Could you check a few things on this model? Use its own coordinates, in mm. A direction names the side the tool comes from. Give positions to 0.01 mm unless a question says otherwise; leave off trailing zeros. Loops run counter-clockwise (first coordinate to the right, second up) from the corner with the lowest first, then second, coordinate; pieces in that order, holes last. Notation, with made-up numbers: (-2, 18.5) -> (29, 18.5) arc R25 ccw to (29, 52.5) -> close; hole circle Ø7 at (25.5, 41.25). An arc over 180 degrees is marked (long way). Write each question's results on one line, items separated by ' | '. Start each with the question number.
Q1. We'd pull the mould along Z, two halves only. Please class faces 5 (the face through (12.446, 88.46, -178.465)), 6 (the face through (196, 87.7, -346.1)), 7 (the face through (-12, 177.8, -108)): released by +Z, released by -Z, zero draft, split by the parting line, or undercut.
Q2. If we section it at C-C, the plane x = 146.05: List the corners of the cut face in (y, z) for me (1 decimal).
Q3. If I drill on line 1 along Z through (x, y) = (146.05, 76) (1 decimal); line 2 along Y through (x, z) = (110, -272); line 3 along Z through (x, y) = (192.5, 96.5), over which ranges is the centre line in solid material (lowest first)?
Q4. Will these pins go through, and if not, where does the flat tip stop? P1, Ø0.8, axis at y = 40.5, z = 5.5, coming from the +X side; P2, Ø1.7, axis at x = -39, y = 40.5, coming from the +Z side (3 decimals); P3, Ø0.7, axis at y = 84, z = -36, coming from the -X side (3 decimals); P4, Ø5, axis at x = 142.5, z = -298, coming from the -Y side.
Q5. Which directions (+Z, -Z, +X, -X, +Y, -Y) give clear straight access to the entire face, cutting with the end or side of a thin tool? Please do faces 1 (the face through (64, 39.688, 25)), 2 (the face through (100, 0, -154)), 3 (the face through (-38.9, 41.275, -23.5)), 4 (the face through (-21.262, 21.153, 38.673)).
Q6. If we section it at D-D, the plane z = -306: List the corners of the cut face in (x, y) for me.
from build123d import *

# Parameters (mm, degrees)
F1_DEPTH  = 177.8
F3_T      = -1.5875
F4_W      = 201.5869445521
F4_H      = 226.8152372871
F5_DEPTH  = 137.796
F6_R      = 3.571875
F7_DEPTH  = 1.5875
F9_W      = 76.2
F9_H      = 19.05
F10_DEPTH = 154.0954613767


with BuildPart() as f1:
    # F0 (on Front) → F1 (new body)
    with BuildSketch(Plane.XZ):
        with BuildLine():
            Line((224.489292991, -184.5372190302), (34.2280551234, 30.3110316959))
            ThreePointArc((34.2280551234, 30.3110316959), (-22.7900998011, 39.6349561758), (-43.415004865, -14.3337277974))
            Line((-43.415004865, -14.3337277974), (46.5572805176, -286.8481262024))
            ThreePointArc((46.5572805176, -286.8481262024), (198.2773120441, -344.8301079029), (224.489292991, -184.5372190302))
        make_face()
    extrude(amount=-F1_DEPTH)

    # F3
    f3_openings = [f1.faces().sort_by_distance(p)[0] for p in [
        (100.456199, 177.8, -174.706432),
    ]]
    offset(amount=F3_T, openings=f3_openings)

    # F4 (on offset) → F5 (cut, through all)
    with BuildSketch(Plane.YZ.offset(92.075)):
        with Locations((142.068472276, 21.3326186436)):
            Rectangle(F4_W, F4_H)
    extrude(amount=-F5_DEPTH, mode=Mode.SUBTRACT)

    # F6 (on face) → F7 (join)
    with BuildSketch(Plane(origin=(0, 41.275, 0), x_dir=(-1, 0, 0), z_dir=(0, 1, 0))):
        with BuildLine():
            Line((-13.52243099, 42.0097776282), (-80.9625, 41.275))
            Line((-80.9625, 41.275), (-80.9625, -24.8573199515))
            Line((-80.9625, -24.8573199515), (-33.0395809871, 29.2585653176))
            ThreePointArc((-33.0395809871, 29.2585653176), (-24.1382185276, 36.9462306949), (-13.52243099, 42.0097776282))
        make_face()
        with Locations((-71.4375, 22.47392)):
            Circle(F6_R, mode=Mode.SUBTRACT)
        with BuildLine():
            Line((80.9625, -73.025), (80.9625, 41.275))
            Line((80.9625, 41.275), (15.6221615422, 41.275))
            ThreePointArc((15.6221615422, 41.275), (39.833691772, 18.9988040694), (41.9075394183, -13.8360289155))
            Line((41.9075394183, -13.8360289155), (22.3659407759, -73.025))
            Line((22.3659407759, -73.025), (80.9625, -73.025))
        make_face()
        with Locations((71.4375, -53.72608)):
            Circle(F6_R, mode=Mode.SUBTRACT)
        with Locations((71.4375, -15.62608)):
            Circle(F6_R, mode=Mode.SUBTRACT)
        with Locations((71.4375, 22.47392)):
            Circle(F6_R, mode=Mode.SUBTRACT)
    extrude(amount=-F7_DEPTH)

    # F9 (on offset) → F10 (cut, up to face)
    with BuildSketch(Plane.YZ.offset(-152.4)):
        with Locations((139.7, -133.35)):
            Rectangle(F9_W, F9_H)
    extrude(amount=F10_DEPTH, mode=Mode.SUBTRACT)


solid = f1.part
Final values:
1) face 5: undercut | face 6: split by the parting line | face 7: zero draft
2) outline: (0, -358.8) -> (177.8, -358.8) -> (177.8, -357.2) -> (1.6, -357.2) -> (1.6, -98.4) -> (177.8, -98.4) -> (177.8, -96) -> (0, -96) -> close
3) line 1: z = -358.8 to -357.2, -98.4 to -96 | line 2: y = 0 to 1.59 | line 3: z = -347.92 to -346.14, -150.81 to -148.41
4) P1: stops at x = 80.96 | P2: stops at z = 41.275 | P3: stops at x = 92.075 | P4: stops at y = 0
5) face 1: +Z, +X, -Y | face 2: +Z, -Z, +X, -X, -Y | face 3: +Z, -X, +Y | face 4: +Y
6) outline: (55.09, 0) -> (237.01, 0) -> (237.01, 177.8) -> (235.18, 177.8) -> (235.18, 1.59) -> (56.92, 1.59) -> (56.92, 177.8) -> (55.09, 177.8) -> close
